Part model, mm, in its own coordinate system. A direction names the side the tool comes from. Coordinates: 2 decimals unless noted, no trailing zeros. Loops run counter-clockwise (first coordinate to the right, second up) from the corner with the lowest first, then second, coordinate; pieces in that order, holes last. Notation, with made-up numbers: (-2.5, 79.25) - (46.5, 79.25) arc R29 ccw to (46.5, 104.25) - close; hole circle Ø6 at (18, 29). An arc over 180 degrees is marked (long way). Answer as CSV lines item,"result".
from build123d import *
from OCP.BRepFilletAPI import BRepFilletAPI_MakeChamfer

# Parameters (mm, degrees)
BOSS_EXTRUDE1_DEPTH           = 38.1
SKETCH2_R                     = 3.1115
CASTER_MOUNT_HOLES_DEPTH      = 159.225945815
SKETCH6_R                     = 1.5875
FRAME_MOUNTHOLES_DEPTH        = 159.636980569
SKETCH7_W                     = 46.99
SKETCH7_H                     = 15.875
LEG_CUTOUTS_DEPTH             = 172.505541744
CHAMFER1_SIZE                 = 1.27
CHAMFER1_SIZE2                = 3.444253967
SKETCH8_R                     = 1.5875
ELECTRONICS_MOUNT_HOLES_DEPTH = 159.225945815
CHAMFER2_SIZE                 = 1.27
CHAMFER2_SIZE2                = 3.444253967
FILLET1_R                     = 3.81
FILLET2_R                     = 3.048
SKETCH9_R                     = 5.715
CUT_EXTRUDE1_DEPTH            = 3.048
SKETCH10_R                    = 3.175
CUT_EXTRUDE2_DEPTH            = 2.159


with BuildPart() as part:
    # Sketch1 → Boss-Extrude1 (new, symmetric)
    with BuildSketch(Plane(origin=(0, 0, 0), x_dir=(0, 0, -1), z_dir=(1, 0, 0))):
        Polygon((-152.4, 0), (-132.001014052, 0), (-121.125726695, 18.923), (-18.574273305, 18.923), (-7.698985948, 0), (12.7, 0), (12.7, 4.445), (0, 4.445), (-12.7, 26.543), (-127, 26.543), (-139.7, 4.445), (-152.4, 4.445), align=None)
    extrude(amount=BOSS_EXTRUDE1_DEPTH, both=True)

    # Sketch2 → Caster-Mount-Holes (cut, through all)
    with BuildSketch(Plane.XZ.offset(-18.923)):
        with Locations(Location((-11.938, 88.138, 0), (0, 0, 270))):
            Circle(SKETCH2_R)
        with Locations(Location((11.938, 88.138, 0), (0, 0, 270))):
            Circle(SKETCH2_R)
        with Locations(Location((11.938, 33.782, 0), (0, 0, 90))):
            Circle(SKETCH2_R)
        with Locations(Location((-11.938, 33.782, 0), (0, 0, 90))):
            Circle(SKETCH2_R)
    extrude(amount=-CASTER_MOUNT_HOLES_DEPTH, mode=Mode.SUBTRACT)

    # Sketch6 → Frame-MountHoles (cut, through all)
    with BuildSketch(Plane(origin=(0, 4.445, 0), x_dir=(1, 0, 0), z_dir=(0, 1, 0))):
        with Locations(Location((-31.115, 6.35, 0), (0, 0, 270))):
            Circle(SKETCH6_R)
        with Locations(Location((31.115, 6.35, 0), (0, 0, 90))):
            Circle(SKETCH6_R)
        with Locations(Location((31.115, -146.05, 0), (0, 0, 270))):
            Circle(SKETCH6_R)
        with Locations(Location((-31.115, -146.05, 0), (0, 0, 90))):
            Circle(SKETCH6_R)
    extrude(amount=-FRAME_MOUNTHOLES_DEPTH, mode=Mode.SUBTRACT)

    # Sketch7 → Leg-Cutouts (cut, through all)
    with BuildSketch(Plane(origin=(0, 0, -12.7), x_dir=(-1, 0, 0), z_dir=(0, 0, -1))):
        with Locations((0, 7.9375)):
            Rectangle(SKETCH7_W, SKETCH7_H)
    extrude(amount=-LEG_CUTOUTS_DEPTH, mode=Mode.SUBTRACT)

    # Chamfer1: one chamfer whose edges measure the first distance from different faces: ONE call of the kernel's chamfer builder (chamfer() names one face for all edges)
    chamfer1_edges_1 = [part.edges().sort_by_distance(p)[0] for p in [
        (30.7975, 0, 7.698985948),
        (-30.7975, 0, 7.698985948),
    ]]
    chamfer1_side_1 = [part.faces().sort_by_distance(p)[0] for p in [
        (0, 18.235769515, 18.179313256),
    ]]
    chamfer1_edges_2 = [part.edges().sort_by_distance(p)[0] for p in [
        (30.7975, 0, 132.001014052),
    ]]
    chamfer1_side_2 = [part.faces().sort_by_distance(p)[0] for p in [
        (30.788832212, 0, 142.09541541),
    ]]
    chamfer1_edges_3 = [part.edges().sort_by_distance(p)[0] for p in [
        (-30.7975, 0, 132.001014052),
    ]]
    chamfer1_side_3 = [part.faces().sort_by_distance(p)[0] for p in [
        (-30.788832212, 0, 142.09541541),
    ]]
    chamfer1 = BRepFilletAPI_MakeChamfer(part.part.solid().wrapped)
    for e in chamfer1_edges_1:
        chamfer1.Add(CHAMFER1_SIZE, CHAMFER1_SIZE2, e.wrapped, chamfer1_side_1[0].wrapped)  # the first distance lies on this face
    for e in chamfer1_edges_2:
        chamfer1.Add(CHAMFER1_SIZE, CHAMFER1_SIZE2, e.wrapped, chamfer1_side_2[0].wrapped)  # the first distance lies on this face
    for e in chamfer1_edges_3:
        chamfer1.Add(CHAMFER1_SIZE, CHAMFER1_SIZE2, e.wrapped, chamfer1_side_3[0].wrapped)  # the first distance lies on this face
    add(Compound.cast(chamfer1.Shape()), mode=Mode.REPLACE)

    # Sketch8 → Electronics-Mount-Holes (cut, through all)
    with BuildSketch(Plane.XZ.offset(-18.923)):
        with Locations(Location((-30.1625, 105.41, 0), (0, 0, 270))):
            Circle(SKETCH8_R)
        with Locations(Location((-30.1625, 67.31, 0), (0, 0, 270))):
            Circle(SKETCH8_R)
        with Locations(Location((30.1625, 67.31, 0), (0, 0, 90))):
            Circle(SKETCH8_R)
        with Locations(Location((30.1625, 105.41, 0), (0, 0, 90))):
            Circle(SKETCH8_R)
    extrude(amount=-ELECTRONICS_MOUNT_HOLES_DEPTH, mode=Mode.SUBTRACT)

    # Chamfer2: one chamfer whose edges measure the first distance from different faces: ONE call of the kernel's chamfer builder (chamfer() names one face for all edges)
    chamfer2_edges_1 = [part.edges().sort_by_distance(p)[0] for p in [
        (0, 26.543, 127),
    ]]
    chamfer2_side_1 = [part.faces().sort_by_distance(p)[0] for p in [
        (0, 26.543, 69.915297007),
    ]]
    chamfer2_edges_2 = [part.edges().sort_by_distance(p)[0] for p in [
        (0, 26.543, 12.7),
    ]]
    chamfer2_side_2 = [part.faces().sort_by_distance(p)[0] for p in [
        (0, 17.992202532, 7.785748581),
    ]]
    chamfer2 = BRepFilletAPI_MakeChamfer(part.part.solid().wrapped)
    for e in chamfer2_edges_1:
        chamfer2.Add(CHAMFER2_SIZE, CHAMFER2_SIZE2, e.wrapped, chamfer2_side_1[0].wrapped)  # the first distance lies on this face
    for e in chamfer2_edges_2:
        chamfer2.Add(CHAMFER2_SIZE, CHAMFER2_SIZE2, e.wrapped, chamfer2_side_2[0].wrapped)  # the first distance lies on this face
    add(Compound.cast(chamfer2.Shape()), mode=Mode.REPLACE)

    # Fillet1
    fillet1_edges = [part.edges().sort_by_distance(p)[0] for p in [
        (0, 18.923, 18.574273305),
        (0, 18.923, 121.125726695),
        (23.495, 15.875, 11.695757342),
        (23.495, 15.875, 128.004242658),
        (-23.495, 15.875, 128.004242658),
        (-23.495, 15.875, 11.695757342),
    ]]
    fillet(fillet1_edges, radius=FILLET1_R)

    # Fillet2
    fillet2_edges = [part.edges().sort_by_distance(p)[0] for p in [
        (30.7975, 4.445, 0),
        (30.7975, 4.445, 139.7),
        (-30.7975, 4.445, 0),
        (-30.7975, 4.445, 139.7),
    ]]
    fillet(fillet2_edges, radius=FILLET2_R)

    # Sketch9 → Cut-Extrude1 (cut)
    with BuildSketch(Plane(origin=(0, 26.543, 0), x_dir=(1, 0, 0), z_dir=(0, 1, 0))):
        with Locations(Location((-11.938, -33.782, 0), (0, 0, 270))):
            Circle(SKETCH9_R)
        with Locations(Location((11.938, -33.782, 0), (0, 0, 270))):
            Circle(SKETCH9_R)
        with Locations(Location((-11.938, -88.138, 0), (0, 0, 270))):
            Circle(SKETCH9_R)
        with Locations(Location((11.938, -88.138, 0), (0, 0, 270))):
            Circle(SKETCH9_R)
    extrude(amount=-CUT_EXTRUDE1_DEPTH, mode=Mode.SUBTRACT)

    # Sketch10 → Cut-Extrude2 (cut)
    with BuildSketch(Plane.XZ.offset(-18.923)):
        with Locations(Location((-30.1625, 105.41, 0), (0, 0, 270))):
            Circle(SKETCH10_R)
        with Locations(Location((-30.1625, 67.31, 0), (0, 0, 270))):
            Circle(SKETCH10_R)
        with Locations(Location((30.1625, 105.41, 0), (0, 0, 270))):
            Circle(SKETCH10_R)
        with Locations(Location((30.1625, 67.31, 0), (0, 0, 270))):
            Circle(SKETCH10_R)
    extrude(amount=-CUT_EXTRUDE2_DEPTH, mode=Mode.SUBTRACT)


solid = part.part
Q1. Flat gauge pins, fed straight in: pin 1 (8 mm diameter, centred on x = 0, y = 21, fed in from +Z); pin 2 (5 mm diameter, centred on x = -9, z = 11, fed in from -Y) (3 decimals); pin 3 (10 mm diameter, centred on x = 26.5, z = 43.5, fed in from -Y); pin 4 (12 mm diameter, centred on x = 0, y = 9, fed in from +Z). Where does each tip first touch, or does it go through?
Results:
pin 1,"stops at z = 132.48"
pin 2,"stops at y = 15.875"
pin 3,"stops at y = 18.92"
pin 4,"passes through"
Q2. Saw through at C-C (x = -25.5). Give the cut face in (y, z) (3 decimals), then the cut area to 3 significant figures.
Results:
outline,"(0, -12.7) - (4.445, -12.7) - (4.445, -1.764) arc R3.048 cw to (5.974, 0.879) - (25.442, 12.067) - (26.543, 16.144) - (26.543, 125.73) - (23.557, 128.716) - (5.974, 138.821) arc R3.048 cw to (4.445, 141.464) - (4.445, 152.4) - (0, 152.4) - (0, 133.271) - (2.986, 130.285) - (17.011, 122.224) arc R3.81 cw to (18.923, 118.921) - (18.923, 20.779) arc R3.81 cw to (17.011, 17.476) - (1.101, 8.332) - (0, 4.255) - close"
area,"1,390 mm^2"
Q3. Saw through at A-A (z = 105.41). Count the separate pieces of the cut face and the enclosed holes in it, then the cut area to 3 significant figures.
Results:
separate pieces,"3"
enclosed holes,"0"
area,"519 mm^2"
Q4. Which spindle directions (+Z, -Z, +X, -X, +Y, -Y) get a long thin tool onto all of the face, cutting with end or side? Do faces 4 (the face through (-14, 23.495, 91)), 5 (the face through (0, 15.875, 128)), 6 (the face through (30.302, 19.987, 108.582)). Say none if no direction does.
Results:
face 4,"+Y"
face 5,"+Z, -Z, -Y"
face 6,"-Y"
Q5. Wall check: L1, parallel to X at y = 3.55, z = 146.05 (1 decimal); L2, parallel to X at y = 25.1, z = 67.31 (3 decimals); L3, parallel to X at y = 19.4, z = 105.41. Give the ranges that are in metal, low to high.
Results:
L1,"x = -38.1 to -32.7, -29.5 to -23.5, 23.5 to 29.5, 32.7 to 38.1"
L2,"x = -38.1 to -31.75, -28.575 to 28.575, 31.75 to 38.1"
L3,"x = -38.1 to -33.34, -26.99 to 26.99, 33.34 to 38.1"
Q6. Saw through at B-B (z = -6.35). Give the cut face in (x, y) (1 decimal), then the cut area to 3 significant figures.
Results:
outline,"(-38.1, 0) - (-32.7, 0) - (-32.7, 4.4) - (-38.1, 4.4) - close; (-29.5, 0) - (-23.5, 0) - (-23.5, 4.4) - (-29.5, 4.4) - close; (23.5, 0) - (29.5, 0) - (29.5, 4.4) - (23.5, 4.4) - close; (32.7, 0) - (38.1, 0) - (38.1, 4.4) - (32.7, 4.4) - close"
area,"102 mm^2"
Q7. Two-plate mould, pull along Z, no slides. Class faces 1 (the face through (31, 2, 152.4)), 2 (the face through (32, 21.082, 105)), 3 (the face through (23.495, 5, 139)): released by +Z, released by -Z, zero draft, split by the parting line, or undercut.
Results:
face 1,"released by +Z"
face 2,"undercut"
face 3,"zero draft"
